Work out the finished part from the listing and answer in its coordinate system (mm). Face numbers are marked on the shaded views. A direction names the side the tool comes from. Round coordinates to 2 decimals unless told otherwise and drop trailing zeros. Order: outer loops, then holes, each group sorted by start corner. A loop starts at its lowest first (then second) coordinate and runs counter-clockwise, first axis right, second up. Notation, with made-up numbers: (20.5, -30.75) -> (39.5, -30.75) arc R18 ccw to (39.5, -6.75) -> close; hole circle Ø1 at (74, 33.25). An arc over 180 degrees is marked (long way). Use a Markdown table: item, result. Add a question column.
Item 1: A cutting plane is placed at B-B, the plane x = 8.5. Determine the outline of the cut face in (y, z), plus the area to 3 significant figures.
Item 2: A cutting plane is placed at C-C, the plane z = 11.25. Give the number of separate pieces and of enclosed holes in the cut face, plus the area to 3 significant figures.
Item 3: Find the intervals of material crossed by L1, parallel to Y at x = 23.3, z = 6.1; L2, parallel to X at y = 33.64, z = 10.7 (3 decimals); L3, parallel to X at y = 18, z = 9.5, in increasing order. Write a range as [from, to].
Item 4: A cutting plane is placed at A-A, the plane y = 30.94. Determine the outline of the cut face in (x, z) (3 decimals), plus the area to 3 significant figures.
Item 5: For a pull along X with two mould halves and no side action, classify the marked faces 1, 2, 3 and 4 as +X half, -X half, draft (parallel to the pull), parting line (faces both ways), or undercut.
Item 6: A flat-ended cylindrical pin translates along its axis: P1, Ø1.6, axis at x = 20.65, y = 30.94, coming from the +Z side. Find the tip coordinate at first contact, or state that the pin passes through.
Item 7: A cutting plane is placed at D-D, the plane x = 1.7. Determine the outline of the cut face in (y, z) (3 decimals).
Item 8: A tool of negligible diameter and unlimited length cuts with its end or side. For the marked faces 5 and 6, from which of +Z, -Z, +X, -X, +Y, -Y can it reach the whole face along a straight path? Write none if from no direction.
from build123d import *

# Parameters (mm, degrees)
SKETCH_1_W           = 25.95
SKETCH_1_H           = 36.24
EXTRUDE_4_DEPTH      = 5
SKETCH_1_4_W         = 25.95
SKETCH_1_4_H         = 36.24
SKETCH_1_4_W_2       = 23.35
SKETCH_1_4_H_2       = 33.64
EXTRUDE_6_DEPTH      = 13
SKETCH_2_W           = 9.2
SKETCH_2_H           = 4
CUT_EXTRUDE_1_DEPTH  = 2
HOLE_WIZARD_M1_6_1_D = 1.25
SKETCH_5_W           = 9.2
SKETCH_5_H           = 6
CUT_EXTRUDE_2_DEPTH  = 0.5
SKETCH_6_R           = 0.8
CUT_EXTRUDE_3_DEPTH  = 46.039050834
M1_2X0_25_1_D        = 0.95
SKETCH_9_R           = 0.8
CUT_EXTRUDE_4_DEPTH  = 2
M1_2X0_25_2_D        = 0.95
M1_2X0_25_2_DEPTH    = 3.15
M1_2X0_25_2_TIP      = 0.285408794
M1_2X0_25_3_D        = 0.95
M1_2X0_25_3_DEPTH    = 3.15
M1_2X0_25_3_TIP      = 0.285408794


with BuildPart() as part:
    # Sketch 1 → Extrude 4 (new body)
    with BuildSketch(Plane.XY):
        with Locations((11.175, 16.32)):
            Rectangle(SKETCH_1_W, SKETCH_1_H)
    extrude(amount=EXTRUDE_4_DEPTH)

    # Sketch 1_4 → Extrude 6 (add)
    with BuildSketch(Plane.XY):
        with Locations((11.175, 16.32)):
            Rectangle(SKETCH_1_4_W, SKETCH_1_4_H)
        with Locations((11.175, 16.32)):
            Rectangle(SKETCH_1_4_W_2, SKETCH_1_4_H_2, mode=Mode.SUBTRACT)
    extrude(amount=EXTRUDE_6_DEPTH)

    # Sketch 2 → Cut-Extrude 1 (cut)
    with BuildSketch(Plane(origin=(0, 34.44, 0), x_dir=(1, 0, 0), z_dir=(0, 1, 0))):
        with Locations((11.07, -7)):
            Rectangle(SKETCH_2_W, SKETCH_2_H)
    extrude(amount=-CUT_EXTRUDE_1_DEPTH, mode=Mode.SUBTRACT)

    # Hole Wizard M1.6 _1 (through all)
    with Locations(Plane.XY.offset(5)):
        with Locations((1.7, 1.7), (20.65, 1.7), (20.65, 30.94), (1.7, 30.94)):
            Hole(HOLE_WIZARD_M1_6_1_D / 2)

    # Sketch 5 → Cut-Extrude 2 (cut)
    with BuildSketch(Plane.XY.offset(5)):
        with Locations((11.07, 30.14)):
            Rectangle(SKETCH_5_W, SKETCH_5_H)
    extrude(amount=-CUT_EXTRUDE_2_DEPTH, mode=Mode.SUBTRACT)

    # Sketch 6 → Cut-Extrude 3 (cut, through all)
    with BuildSketch(Plane(origin=(24.15, 0, 0), x_dir=(0, 0, -1), z_dir=(1, 0, 0))):
        with Locations((-6.1, 9.168)):
            Circle(SKETCH_6_R)
    extrude(amount=-CUT_EXTRUDE_3_DEPTH, mode=Mode.SUBTRACT)

    # M1.2x0.25 _1 (through all)
    with Locations(Plane(origin=(24.15, 15.218, 6.1), x_dir=(0, 0, 1), z_dir=(1, 0, 0))):
        with Locations((0, 0), (0, 12.1)):
            Hole(M1_2X0_25_1_D / 2)

    # Sketch 9 → Cut-Extrude 4 (cut)
    with BuildSketch(Plane.XZ.offset(1.8)):
        with Locations(Location((7.166, 6.1, 0), (0, 0, 270))):
            Circle(SKETCH_9_R)
        with Locations(Location((15.166, 6.1, 0), (0, 0, 270))):
            Circle(SKETCH_9_R)
    extrude(amount=-CUT_EXTRUDE_4_DEPTH, mode=Mode.SUBTRACT)

    # M1.2x0.25 _2
    with Locations(Plane(origin=(4.141, -1.8, 0.860546307), x_dir=(0, 0, -1), z_dir=(0, -1, 0))):
        with Locations((0, 0), (-10.478907386, 6.05), (0, 8), (-10.478907386, 14.05)):
            Hole(M1_2X0_25_2_D / 2, depth=M1_2X0_25_2_DEPTH)
            with Locations((0, 0, -(M1_2X0_25_2_DEPTH + M1_2X0_25_2_TIP / 2))):  # 118° drill point
                Cone(0, M1_2X0_25_2_D / 2, M1_2X0_25_2_TIP, mode=Mode.SUBTRACT)

    # M1.2x0.25 _3
    with Locations(Plane(origin=(-1, 33.64, 13), x_dir=(1, 0, 0), z_dir=(0, 0, 1))):
        with Locations((0, 0), (24.35, 0), (0, -34.64), (24.35, -34.64)):
            Hole(M1_2X0_25_3_D / 2, depth=M1_2X0_25_3_DEPTH)
            with Locations((0, 0, -(M1_2X0_25_3_DEPTH + M1_2X0_25_3_TIP / 2))):  # 118° drill point
                Cone(0, M1_2X0_25_3_D / 2, M1_2X0_25_3_TIP, mode=Mode.SUBTRACT)


solid = part.part
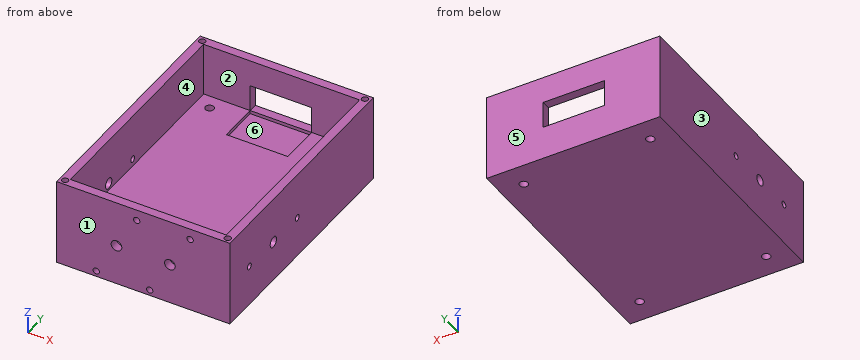
Reported:
| question | item | result |
|---|---|---|
| 1 | outline | (-1.8, 0) -> (34.44, 0) -> (34.44, 5) -> (33.14, 5) -> (33.14, 4.5) -> (27.14, 4.5) -> (27.14, 5) -> (-0.5, 5) -> (-0.5, 13) -> (-1.8, 13) -> close; (33.14, 9) -> (34.44, 9) -> (34.44, 13) -> (33.14, 13) -> close |
| 1 | area | 194 mm² |
| 2 | separate pieces | 2 |
| 2 | enclosed holes | 4 |
| 2 | area | 150 mm² |
| 3 | L1 | [-1.8, 2.64], [3.59, 8.37], [9.97, 14.74], [15.69, 34.44] |
| 3 | L2 | [-1.8, -1.475], [-0.525, 22.875], [23.825, 24.15] |
| 3 | L3 | [-1.8, -0.5], [22.85, 24.15] |
| 4 | outline | (-1.8, 0) -> (1.075, 0) -> (1.075, 5) -> (-0.5, 5) -> (-0.5, 13) -> (-1.8, 13) -> close; (2.325, 0) -> (20.025, 0) -> (20.025, 5) -> (15.67, 5) -> (15.67, 4.5) -> (6.47, 4.5) -> (6.47, 5) -> (2.325, 5) -> close; (21.275, 0) -> (24.15, 0) -> (24.15, 13) -> (22.85, 13) -> (22.85, 5) -> (21.275, 5) -> close |
| 4 | area | 133 mm² |
| 5 | face 1 | draft |
| 5 | face 2 | undercut |
| 5 | face 3 | -X half |
| 5 | face 4 | undercut |
| 6 | P1 | z = 5 |
| 7 | outline | (-1.8, 0) -> (1.075, 0) -> (1.075, 5) -> (-0.5, 5) -> (-0.5, 13) -> (-1.8, 13) -> close; (2.325, 0) -> (30.315, 0) -> (30.315, 5) -> (2.325, 5) -> close; (31.565, 0) -> (34.44, 0) -> (34.44, 13) -> (33.14, 13) -> (33.14, 5) -> (31.565, 5) -> close |
| 8 | face 5 | +Z, -Z, +X, -X, +Y |
| 8 | face 6 | +Z |
